Model file for the job. Use its own axes, mm. A direction names the side the tool comes from. Round coordinates to 2 decimals unless told otherwise and drop trailing zeros. Loops run counter-clockwise (first coordinate to the right, second up) from the corner with the lowest first, then second, coordinate; pieces in that order, holes last. Notation, with made-up numbers: (87.25, 26.5) - (122.25, 26.5) arc R26 ccw to (122.25, 52.5) - close; hole circle Ø4 at (65, 30). An arc over 180 degrees is marked (long way). Answer as a JSON object with one key per item and string values.
from build123d import *

# Parameters (mm, degrees)
F0_W = 5.08
F0_H = 6.604


with BuildPart() as f1:
    # F0 (on Front) → F1 (revolve)
    with BuildSketch(Plane.XZ):
        with Locations((3.215322, 12.7)):
            Rectangle(F0_W, F0_H)
        with BuildLine():
            Line((-4.404678, 25.527), (-4.404678, 19.868769))
            Line((-4.404678, 19.868769), (0.675322, 18.863278))
            Line((0.675322, 18.863278), (0.675322, 16.002))
            Line((0.675322, 16.002), (5.755322, 16.002))
            Line((5.755322, 16.002), (5.755322, 25.527))
            ThreePointArc((5.755322, 25.527), (4.825386, 27.772064), (2.580322, 28.702))
            Line((2.580322, 28.702), (-1.229678, 28.702))
            ThreePointArc((-1.229678, 28.702), (-3.474742, 27.772064), (-4.404678, 25.527))
        make_face()
        Polygon((-4.404678, 6.513816), (-4.404678, 0), (5.755322, 0), (5.755322, 9.398), (0.675322, 9.398), (0.675322, 7.781735), align=None)
    revolve(axis=Axis((0.675322, 0, 0), (1, 0, 0)))


solid = f1.part
1) Drop flat-ended pins along their axis: P1, Ø4, axis at y = -2, z = 14.5, coming from the -X side; P2, Ø4, axis at x = -3, y = 4.5, coming from the +Z side; P3, Ø1.5, axis at x = -3, z = 21.5, coming from the +Y side; P4, Ø1.5, axis at y = -21.5, z = 22.5, coming from the +X side. Give the stop position or say it passes through.
Values follow:
{"P1": "x = 0.68", "P2": "z = 28.52", "P3": "y = 19.25", "P4": "through"}
2) Probe probe 1 along Y at (x, z) = (-0.5, 5.5); probe 2 along Y at (x, z) = (-1.75, -5); probe 3 along Z at (x, y) = (-0.75, -3). List the from-to ranges inside material, lowest first.
Values follow:
{"probe 1": "-28.17 to -18.29, -5.08 to 5.08, 18.29 to 28.17", "probe 2": "-28.22 to -18.69, -5.15 to 5.15, 18.69 to 28.22", "probe 3": "-28.54 to -18.91, -6.79 to 6.79, 18.91 to 28.54"}
3) Tool access for faces 1 (the flat face through (0.675, 0, 8)), 2 (the flat face through (-4.405, 0, 0)): list every direction of +Z, -Z, +X, -X, +Y, -Y with a clear straight run to the whole face (end or side of a thin tool).
Values follow:
{"face 1": "-X", "face 2": "+Z, -Z, -X, +Y, -Y"}
4) Slice it at A-A on y = 0. List the corners of the cut face in (x, z) (3 decimals), then the cut area to 3 significant figures.
Values follow:
{"outline": "(-4.405, -25.527) arc R3.175 ccw to (-1.23, -28.702) - (2.58, -28.702) arc R3.175 ccw to (5.755, -25.527) - (5.755, 25.527) arc R3.175 ccw to (2.58, 28.702) - (-1.23, 28.702) arc R3.175 ccw to (-4.405, 25.527) - (-4.405, 19.869) - (0.675, 18.863) - (0.675, 7.782) - (-4.405, 6.514) - (-4.405, -6.514) - (0.675, -7.782) - (0.675, -18.863) - (-4.405, -19.869) - close", "area": "450 mm²"}
5) Slice it at B-B on x = -3.25. List the corners of the cut face in (y, z).
Values follow:
{"outline": "circle Ø55.95 at (0, 0); circle Ø13.6 at (0, 0); hole circle Ø39.28 at (0, 0)"}
6) Two-plate mould, pull along Y, no slides. Class faces 3 (the flat face through (-4.405, 13.1, -15.2)), 4 (the cylindrical face through (0.65, 28.02, -6.22)), 5 (the conical face through (0.43, -5.68, 18.04)): pulls with the +Y half, pulls with the -Y half, needs draft (parallel to the pull), parting line crosses it, or undercut.
Values follow:
{"face 3": "needs draft", "face 4": "parting line crosses it", "face 5": "undercut"}
